from build123d import *

# Parameters (mm, degrees)
BOSS_EXTRUDE1_DEPTH      = 7.5
BOSS_EXTRUDE1_DEPTH_BACK = 7.5
SKETCH1_R                = 2.25
SKETCH1_R_2              = 1.65
SKETCH2_W                = 8.2
SKETCH2_H                = 5.5
CUT_EXTRUDE1_DEPTH       = 71.61765006
SKETCH2_5_W              = 14
SKETCH2_5_H              = 5.5
CUT_EXTRUDE7_DEPTH       = 14
CUT_EXTRUDE8_START       = -29
SKETCH5_W                = 38.5
SKETCH5_H                = 5.5
CUT_EXTRUDE8_DEPTH       = 8
CUT_EXTRUDE4_START       = 2
SKETCH4_W                = 8
SKETCH4_H                = 5.5
CUT_EXTRUDE4_DEPTH       = 69.61765006
CUT_EXTRUDE5_START       = -2.75
SKETCH1_3_W              = 8.5
SKETCH1_3_H              = 15
SKETCH1_3_R              = 2.25
SKETCH1_3_H_2            = 8.5
CUT_EXTRUDE5_DEPTH       = 68.86765006
CUT_EXTRUDE6_DEPTH       = 71.61765006
CUT_EXTRUDE6_DEPTH_BACK  = 71.61765006
SKETCH1_4_R              = 2.25
CUT_EXTRUDE9_START       = 4.5
SKETCH1_5_R              = 2.9
SKETCH1_5_R_2            = 1.65
CUT_EXTRUDE9_DEPTH       = 3
CUT_EXTRUDE10_START      = -7.5
CUT_EXTRUDE10_DEPTH      = 2.2


with BuildPart() as part:
    # Sketch1 → Boss-Extrude1 (new, two sides: drawn at the far end of the back side and taken through both)
    with BuildSketch(Plane(origin=(0, 0, 0), x_dir=(1, 0, 0), z_dir=(0, 1, 0)).offset(-BOSS_EXTRUDE1_DEPTH_BACK)):
        with BuildLine():
            Line((-15, 33), (6.15, 33))
            ThreePointArc((6.15, 33), (10.15, 37), (6.15, 41))
            Line((6.15, 41), (0, 41))
            Line((0, 41), (0, 45.25))
            Line((0, 45.25), (-7.5, 45.25))
            ThreePointArc((-7.5, 45.25), (-8.217662602, 45.367522476), (-8.860354994, 45.707812987))
            Line((-8.860354994, 45.707812987), (-13, 48.85))
            Line((-13, 48.85), (-13, 55.75))
            Line((-13, 55.75), (-21, 55.75))
            Line((-21, 55.75), (-21, 59.95))
            ThreePointArc((-21, 59.95), (-25, 63.95), (-29, 59.95))
            Line((-29, 59.95), (-29, 0))
            Line((-29, 0), (-15, 0))
            Line((-15, 0), (-15, 33))
        make_face()
        with Locations(Location((-19.25, 20.25, 0), (0, 0, 270))):
            Circle(SKETCH1_R, mode=Mode.SUBTRACT)
        with Locations(Location((-16.5, 51.75, 0), (0, 0, 270))):
            Circle(SKETCH1_R_2, mode=Mode.SUBTRACT)
        with Locations(Location((-25, 59.95, 0), (0, 0, 270))):
            Circle(SKETCH1_R_2, mode=Mode.SUBTRACT)
        with Locations(Location((6.15, 37, 0), (0, 0, 270))):
            Circle(SKETCH1_R_2, mode=Mode.SUBTRACT)
    extrude(amount=BOSS_EXTRUDE1_DEPTH + BOSS_EXTRUDE1_DEPTH_BACK)

    # Sketch2 → Cut-Extrude1 (cut, through all)
    with BuildSketch(Plane(origin=(0, 0, 0), x_dir=(0, 0, -1), z_dir=(1, 0, 0))):
        with Locations((59.85, 0)):
            Rectangle(SKETCH2_W, SKETCH2_H)
    extrude(amount=-CUT_EXTRUDE1_DEPTH, mode=Mode.SUBTRACT)

    # Sketch2<5> → Cut-Extrude7 (cut)
    with BuildSketch(Plane(origin=(0, 0, 0), x_dir=(0, 0, -1), z_dir=(1, 0, 0))):
        with Locations((48, 0)):
            Rectangle(SKETCH2_5_W, SKETCH2_5_H)
    extrude(amount=-CUT_EXTRUDE7_DEPTH, mode=Mode.SUBTRACT)

    # Sketch5 → Cut-Extrude8 (cut)
    with BuildSketch(Plane(origin=(0, 0, 0), x_dir=(0, 0, -1), z_dir=(1, 0, 0)).offset(CUT_EXTRUDE8_START)):
        with Locations((44.7, 0)):
            Rectangle(SKETCH5_W, SKETCH5_H)
    extrude(amount=CUT_EXTRUDE8_DEPTH, mode=Mode.SUBTRACT)

    # Sketch4 → Cut-Extrude4 (cut, through all)
    with BuildSketch(Plane(origin=(0, 0, 0), x_dir=(0, 0, -1), z_dir=(1, 0, 0)).offset(CUT_EXTRUDE4_START)):
        with Locations((37, 0)):
            Rectangle(SKETCH4_W, SKETCH4_H)
    extrude(amount=CUT_EXTRUDE4_DEPTH, mode=Mode.SUBTRACT)

    # Sketch1<3> → Cut-Extrude5 (cut, through all)
    # profile 1 of 3: a face of its own
    with BuildSketch(Plane(origin=(0, 0, 0), x_dir=(1, 0, 0), z_dir=(0, 1, 0)).offset(CUT_EXTRUDE5_START)):
        with Locations((-24.75, 7.5)):
            Rectangle(SKETCH1_3_W, SKETCH1_3_H)
        with Locations((-24.75, 10)):
            Circle(SKETCH1_3_R, mode=Mode.SUBTRACT)
    # profile 2 of 3: a face of its own
    with BuildSketch(Plane(origin=(0, 0, 0), x_dir=(1, 0, 0), z_dir=(0, 1, 0)).offset(CUT_EXTRUDE5_START)):
        with Locations((-24.75, 10)):
            Circle(SKETCH1_3_R)
    # profile 3 of 3: a face of its own
    with BuildSketch(Plane(origin=(0, 0, 0), x_dir=(1, 0, 0), z_dir=(0, 1, 0)).offset(CUT_EXTRUDE5_START)):
        with Locations((-19.25, 20.25)):
            Rectangle(SKETCH1_3_W, SKETCH1_3_H_2)
        with Locations(Location((-19.25, 20.25, 0), (0, 0, 270))):
            Circle(SKETCH1_3_R, mode=Mode.SUBTRACT)
    cut_extrude5 = extrude(amount=-CUT_EXTRUDE5_DEPTH, mode=Mode.SUBTRACT)

    # Mirror2: Cut-Extrude5 across plane
    add(cut_extrude5.mirror(Plane.ZX), mode=Mode.SUBTRACT)

    # Sketch1<4> → Cut-Extrude6 (cut, two sides: drawn at the far end of the back side and taken through both)
    with BuildSketch(Plane(origin=(0, 0, 0), x_dir=(1, 0, 0), z_dir=(0, 1, 0)).offset(-CUT_EXTRUDE6_DEPTH_BACK)):
        with Locations(Location((-24.75, 10, 0), (0, 0, 270))):
            Circle(SKETCH1_4_R)
    extrude(amount=CUT_EXTRUDE6_DEPTH + CUT_EXTRUDE6_DEPTH_BACK, mode=Mode.SUBTRACT)

    # Sketch1<5> → Cut-Extrude9 (cut)
    # profile 1 of 4: a face of its own
    with BuildSketch(Plane(origin=(0, 0, 0), x_dir=(1, 0, 0), z_dir=(0, 1, 0)).offset(CUT_EXTRUDE9_START)):
        with Locations(Location((-25, 59.95, 0), (0, 0, 270))):
            Circle(SKETCH1_5_R)
        with Locations(Location((-25, 59.95, 0), (0, 0, 270))):
            Circle(SKETCH1_5_R_2, mode=Mode.SUBTRACT)
    # profile 2 of 4: a face of its own
    with BuildSketch(Plane(origin=(0, 0, 0), x_dir=(1, 0, 0), z_dir=(0, 1, 0)).offset(CUT_EXTRUDE9_START)):
        with Locations((-16.5, 51.75)):
            Circle(SKETCH1_5_R)
        with Locations(Location((-16.5, 51.75, 0), (0, 0, 270))):
            Circle(SKETCH1_5_R_2, mode=Mode.SUBTRACT)
    # profile 3 of 4: a face of its own
    with BuildSketch(Plane(origin=(0, 0, 0), x_dir=(1, 0, 0), z_dir=(0, 1, 0)).offset(CUT_EXTRUDE9_START)):
        with Locations(Location((6.15, 37, 0), (0, 0, 270))):
            Circle(SKETCH1_5_R)
        with Locations(Location((6.15, 37, 0), (0, 0, 270))):
            Circle(SKETCH1_5_R_2, mode=Mode.SUBTRACT)
    # profile 4 of 4: a face of its own
    with BuildSketch(Plane(origin=(0, 0, 0), x_dir=(1, 0, 0), z_dir=(0, 1, 0)).offset(CUT_EXTRUDE9_START)):
        with BuildLine():
            Line((-16.5, 48.85), (-13, 48.85))
            Line((-13, 48.85), (-13, 52.75))
            Line((-13, 52.75), (-13, 55.75))
            Line((-13, 55.75), (-19.4, 55.75))
            Line((-19.4, 55.75), (-19.4, 51.75))
            ThreePointArc((-19.4, 51.75), (-16.5, 54.65), (-13.6, 51.75))
            ThreePointArc((-13.6, 51.75), (-14.449390335, 49.699390335), (-16.5, 48.85))
        make_face()
    extrude(amount=CUT_EXTRUDE9_DEPTH, mode=Mode.SUBTRACT)

    # Sketch6 → Cut-Extrude10 (cut)
    with BuildSketch(Plane(origin=(0, 0, 0), x_dir=(1, 0, 0), z_dir=(0, 1, 0)).offset(CUT_EXTRUDE10_START)):
        Polygon((-21.651368439, 59.95), (-23.325684219, 62.85), (-26.674315781, 62.85), (-28.348631561, 59.95), (-26.674315781, 57.05), (-23.325684219, 57.05), align=None)
        Polygon((-13.151368439, 51.75), (-14.825684219, 54.65), (-18.174315781, 54.65), (-19.848631561, 51.75), (-18.174315781, 48.85), (-14.825684219, 48.85), align=None)
        Polygon((9.498631561, 37), (7.824315781, 39.9), (4.475684219, 39.9), (2.801368439, 37), (4.475684219, 34.1), (7.824315781, 34.1), align=None)
    extrude(amount=CUT_EXTRUDE10_DEPTH, mode=Mode.SUBTRACT)

    # Mirror3: part across plane


with BuildPart() as part_1:
    add(part.part)
    add(part.part.mirror(Plane.XY))


solid = part_1.part
The listing builds one solid part. Answer for the finished solid, in the listing's coordinates (mm). A direction names the side the tool comes from. Round coordinates to 2 decimals unless told otherwise and drop trailing zeros. Order: outer loops, then holes, each group sorted by start corner. A loop starts at its lowest first (then second) coordinate and runs counter-clockwise, first axis right, second up. Notation, with made-up numbers: (17, -3.75) -> (66, -3.75) arc R25 ccw to (66, 35.25) -> close; hole circle Ø7 at (24, 54). An arc over 180 degrees is marked (long way). Put each result on its own line as item: value.
Q1. Section A-A, the plane z = 20.25 is taken. Write down the section's boundary in (x, y), and give its area (4 significant figures).
Results list:
outline: (-29, -7.5) -> (-23.5, -7.5) -> (-23.5, -2.75) -> (-21.5, -2.75) -> (-21.5, 2.75) -> (-23.5, 2.75) -> (-23.5, 7.5) -> (-29, 7.5) -> close; (-17, -2.75) -> (-15, -2.75) -> (-15, 2.75) -> (-17, 2.75) -> close
area: 104.5 mm^2
Q2. Consider line 1 along Z through (x, y) = (-24.75, -1.45); line 2 along Z through (x, y) = (-25, 3.4); line 3 along Z through (x, y) = (-16.5, -2). Determine where each line is inside the solid, lowest interval first.
Results list:
line 1: -25.45 to -12.25, -7.75 to 7.75, 12.25 to 25.45
line 2: -63.95 to -61.6, -58.3 to -15, 15 to 58.3, 61.6 to 63.95
line 3: -55.75 to -53.4, -50.1 to 50.1, 53.4 to 55.75
Q3. Section B-B, the plane x = -3 is taken. Write down the section's boundary in (y, z).
Results list:
outline: (-7.5, -45.25) -> (-2.75, -45.25) -> (-2.75, -41) -> (2.75, -41) -> (2.75, -45.25) -> (7.5, -45.25) -> (7.5, -33) -> (-7.5, -33) -> close; (-7.5, 33) -> (7.5, 33) -> (7.5, 45.25) -> (2.75, 45.25) -> (2.75, 41) -> (-2.75, 41) -> (-2.75, 45.25) -> (-7.5, 45.25) -> close
Q4. Section D-D, the plane y = 6.25 is taken. Count the separate pieces of the cut face and the enclosed holes in it, and give its area (3 significant figures).
Results list:
separate pieces: 1
enclosed holes: 4
area: 1,660 mm^2
Q5. Each of these flat-tipped pins is pushed along its axis until it touches: P1, Ø2.5, axis at x = -21.5, y = -5.5, coming from the +Z side; P2, Ø1.1, axis at x = 5.5, y = -6.5, coming from the -Z side; P3, Ø1, axis at x = 5.5, y = 5, coming from the +Z side. Where does it stop, or does it pass through?
Results list:
P1: z = 63.26
P2: z = -41
P3: z = 41
Q6. Section C-C, the plane y = -0.5 is taken. Write down the section's boundary in (x, z).
Results list:
outline: (-29, -25.45) -> (-21, -25.45) -> (-21, -55.75) -> (-13, -55.75) -> (-13, -55) -> (-14, -55) -> (-14, -41) -> (2, -41) -> (2, -33) -> (-15, -33) -> (-15, 33) -> (2, 33) -> (2, 41) -> (-14, 41) -> (-14, 55) -> (-13, 55) -> (-13, 55.75) -> (-21, 55.75) -> (-21, 25.45) -> (-29, 25.45) -> close; hole circle Ø4.5 at (-24.75, -10); hole circle Ø4.5 at (-24.75, 10); hole circle Ø4.5 at (-19.25, -20.25); hole circle Ø4.5 at (-19.25, 20.25); hole circle Ø3.3 at (-16.5, -51.75); hole circle Ø3.3 at (-16.5, 51.75)
Q7. Determine the mould class of faces 6 (the flat face through (-18, -7.5, 0)), 7 (the flat face through (-19, 5, 24.5)), 8 (the cylindrical face through (-24.91, 5.09, 63.95)) for opening direction Z: pulls with the +Z half, pulls with the -Z half, needs draft (parallel to the pull), parting line crosses it, or undercut.
Results list:
face 6: needs draft
face 7: undercut
face 8: pulls with the +Z half
Q8. Which of the six approach directions +Z, -Z, +X, -X, +Y, -Y give full straight-line access (tool end or side, diameter ignored) to faces 1 (the flat face through (-25, 4.5, -58)), 2 (the flat face through (-23.5, -5, 20)), 3 (the flat face through (-25, -5, -15)), 4 (the flat face through (4, -2.75, 37)), 5 (the flat face through (-22.5, -6.42, -58.48))?
Results list:
face 1: +Y
face 2: +X, -Y
face 3: -X, -Y
face 4: +Z, -Z, +X
face 5: -Y
